```python
from build123d import *

# Parameters (mm, degrees)
SKETCH1_R           = 140
BOSS_EXTRUDE1_DEPTH = 60
SKETCH2_W           = 80
SKETCH2_H           = 80
BOSS_EXTRUDE2_DEPTH = 600
SKETCH3_W           = 180
SKETCH3_H           = 275
BOSS_EXTRUDE3_DEPTH = 230
CUT_EXTRUDE1_DEPTH  = 930.838695689
SKETCH5_W           = 100
SKETCH5_H           = 170
CUT_EXTRUDE2_DEPTH  = 30
SKETCH6_W           = 140
SKETCH6_H           = 210
CUT_EXTRUDE3_DEPTH  = 15
FILLET1_R           = 20
FILLET2_R           = 20
FILLET3_R           = 20


with BuildPart() as part:
    # Sketch1 → Boss-Extrude1 (new body)
    with BuildSketch(Plane(origin=(0, 0, 0), x_dir=(1, 0, 0), z_dir=(0, 1, 0))):
        with Locations(Location((0, 0, 0), (0, 0, 270))):
            Circle(SKETCH1_R)
    extrude(amount=BOSS_EXTRUDE1_DEPTH)

    # Sketch2 → Boss-Extrude2 (add)
    with BuildSketch(Plane(origin=(0, 60, 0), x_dir=(1, 0, 0), z_dir=(0, 1, 0))):
        Rectangle(SKETCH2_W, SKETCH2_H)
    extrude(amount=BOSS_EXTRUDE2_DEPTH)

    # Sketch3 → Boss-Extrude3 (add)
    with BuildSketch(Plane(origin=(0, 660, 0), x_dir=(1, 0, 0), z_dir=(0, 1, 0))):
        Rectangle(SKETCH3_W, SKETCH3_H)
    extrude(amount=BOSS_EXTRUDE3_DEPTH)

    # Sketch4 → Cut-Extrude1 (cut, through all)
    with BuildSketch(Plane.ZY.offset(90)):
        Polygon((22.5, 890), (137.5, 660), (137.5, 890), align=None)
    extrude(amount=-CUT_EXTRUDE1_DEPTH, mode=Mode.SUBTRACT)

    # Sketch5 → Cut-Extrude2 (cut)
    with BuildSketch(Plane(origin=(0, 187, 374), x_dir=(1, 0, 0), z_dir=(0, 0.4472135954999582, 0.8944271909999159))):
        with Locations((0, 657.427894091)):
            Rectangle(SKETCH5_W, SKETCH5_H)
    extrude(amount=-CUT_EXTRUDE2_DEPTH, mode=Mode.SUBTRACT)

    # Sketch6 → Cut-Extrude3 (cut)
    with BuildSketch(Plane(origin=(0, 173.583592135, 347.16718427), x_dir=(1, 0, 0), z_dir=(0, 0.44721359549995826, 0.8944271909999159))):
        with Locations((0, 657.427894091)):
            Rectangle(SKETCH6_W, SKETCH6_H)
    extrude(amount=-CUT_EXTRUDE3_DEPTH, mode=Mode.SUBTRACT)

    # Fillet1
    fillet1_edges = [part.edges().sort_by_distance(p)[0] for p in [
        (0, 60, -140),
        (40, 360, 40),
        (40, 360, -40),
        (-40, 360, -40),
    ]]
    fillet(fillet1_edges, radius=FILLET1_R)

    # Fillet2
    fillet2_edges = [part.edges().sort_by_distance(p)[0] for p in [
        (-40, 360, 40),
    ]]
    fillet(fillet2_edges, radius=FILLET2_R)

    # Fillet3
    fillet3_edges = [part.edges().sort_by_distance(p)[0] for p in [
        (90, 660, 0),
        (0, 660, -137.5),
        (90, 775, -137.5),
        (-90, 660, 0),
        (-90, 775, -137.5),
        (0, 660, 137.5),
        (0, 890, -137.5),
        (-90, 890, -57.5),
        (90, 890, -57.5),
        (0, 890, 22.5),
        (90, 775, 80),
        (-90, 775, 80),
    ]]
    fillet(fillet3_edges, radius=FILLET3_R)


solid = part.part
```
Read the model definition and answer for the solid it produces. Units are mm, in the model's axes. A direction names the side the tool comes from. Give positions to 0.01 mm unless a question says otherwise; leave off trailing zeros. Write each loop counter-clockwise with the first axis right and the second up, starting at its lowest first coordinate (ties: lowest second). Pieces come first, ordered by that corner, then holes. Notation, with made-up numbers: (-18, 81.25) - (26, 81.25) arc R19 ccw to (26, 111.25) - close; hole circle Ø9 at (76.25, -5). An arc over 180 degrees is marked (long way). Write item = value, one per line. Start each with the question number.
Item 1: Find the intervals of material crossed by probe 1 along Y at (x, z) = (-57.5, -88); probe 2 along X at (y, z) = (738, -90); probe 3 along Y at (x, z) = (8, -122), in increasing order. Write a range as [from, to].
Item 2: Each of these flat-tipped pins is pushed along its axis until it touches: P1, Ø1, axis at x = -57, z = 89.5, coming from the +Y side; P2, Ø2, axis at x = 28, y = 532, coming from the -Z side (3 decimals); P3, Ø12, axis at y = 285.5, z = 5.5, coming from the -X side. Where does it stop, or does it pass through?
Item 3: Find section A-A (x = 0). Give the vertices of the cut face in (y, z).
Item 4: Find section B-B (y = 561). Give the vertices of the cut face in (x, z).
Item 5: The mould has two halves that part along Y. Classify faces 4 (the flat face through (-63.2, 762.92, 52.5)), 5 (the flat face through (-1, 890, -55)), 6 (the flat face through (50, 767, 67)), 7 (the flat face through (-1, 774, -137.5)): +Y half, -Y half, draft (parallel to the pull), parting line (faces both ways), or undercut.
Item 6: A tool of negligible diameter and unlimited length cuts with its end or side. For faces 1 (the flat face through (-0.98, 756.212, 39.083)), 2 (the cylindrical face through (33.986, 364.2, 34.297)), 3 (the flat face through (0, 356, -40)), from which of +Z, -Z, +X, -X, +Y, -Y can it reach the whole face along a straight path? Write none if from no direction.
Response:
q1.probe_1 = [0, 60], [660, 890]
q1.probe_2 = [-90, 90]
q1.probe_3 = [0, 59.87], [660.51, 889.49]
q2.P1 = 757
q2.P2 = -38.735
q2.P3 = -40
q3.outline = (0, -140) - (40, -140) arc R20 ccw to (60, -120) - (60, -40) - (660, -40) - (660, -117.5) arc R20 ccw to (680, -137.5) - (870, -137.5) arc R20 ccw to (890, -117.5) - (890, 10.14) arc R20 ccw to (878.94, 28.03) - (851.05, 41.98) - (837.63, 15.14) - (855.52, 6.2) - (848.81, -7.22) - (660.98, 86.7) - (667.69, 100.11) - (685.58, 91.17) - (699, 118) - (688.94, 123.03) arc R20 ccw to (660, 105.14) - (660, 40) - (60, 40) - (60, 120) arc R20 ccw to (40, 140) - (0, 140) - close
q4.outline = (-40, -20) arc R20 ccw to (-20, -40) - (20, -40) arc R20 ccw to (40, -20) - (40, 20) arc R20 ccw to (20, 40) - (-20, 40) arc R20 ccw to (-40, 20) - close
q5.face_4 = undercut
q5.face_5 = +Y half
q5.face_6 = undercut
q5.face_7 = draft
q6.face_1 = none
q6.face_2 = +Z, +X
q6.face_3 = -Z, +X, -X
